For this review, take the finished solid that the model builds, in its own axes (mm). Round coordinates to 2 decimals unless told otherwise and drop trailing zeros. Order: outer loops, then holes, each group sorted by start corner. A loop starts at its lowest first (then second) coordinate and runs counter-clockwise, first axis right, second up. Notation, with made-up numbers: (83, 76) - (101, 76) arc R33 cw to (101, 114) - close; hole circle Ø4 at (-16, -25). An arc over 180 degrees is marked (long way). One line per question, with ' | ' between items.
```python
from build123d import *

# Parameters (mm, degrees)
CUT_EXTRUDE1_DEPTH = 0.8


with BuildPart() as part:
    # Sketch2 → Revolve1 (revolve)
    with BuildSketch(Plane.XY, mode=Mode.PRIVATE) as revolve1_sk:
        Polygon((0, 0), (0, 3), (0.2, 3), (1.7, 1.5), (17.75, 1.5), (18, 1.25), (18, 0), align=None)
    revolve(revolve1_sk.sketch.rotate(Axis((-2.281841559, 0, 0), (1, 0, 0)), 90), axis=Axis((-2.281841559, 0, 0), (1, 0, 0)))

    # Sketch3 → Cut-Extrude1 (cut)
    with BuildSketch(Plane.ZY):
        Polygon((0.721687836, -1.25), (1.443375673, 0), (0.721687836, 1.25), (-0.721687836, 1.25), (-1.443375673, 0), (-0.721687836, -1.25), align=None)
    extrude(amount=-CUT_EXTRUDE1_DEPTH, mode=Mode.SUBTRACT)


solid = part.part
```
(1) We need section B-B on x = 9.25. State the section outline as (y, z) points.
Output values:
outline: circle Ø3 at (0, 0)
(2) We need section A-A on z = 0. State the section outline as (x, y) points, plus the area to 3 significant figures.
Output values:
outline: (0, -3) - (0.2, -3) - (1.7, -1.5) - (17.75, -1.5) - (18, -1.25) - (18, 1.25) - (17.75, 1.5) - (1.7, 1.5) - (0.2, 3) - (0, 3) - (0, 1.25) - (0.8, 1.25) - (0.8, -1.25) - (0, -1.25) - close | area: 54.8 mm^2
(3) Mouldability with a two-part tool opening along Z and no side actions: class faces 1 (the flat face through (0, 0.6, -1.3)), 2 (the flat face through (0.8, 0, 0)), 3 (the cylindrical face through (9.84, -0.45, 1.43)) as released by +Z, released by -Z, zero draft, split by the parting line, or undercut.
Output values:
face 1: zero draft | face 2: undercut | face 3: split by the parting line
(4) Insertion check: pin 1 (3 mm diameter, centred on x = 16, z = 1.5, fed in from -Y); pin 2 (3 mm diameter, centred on x = 10, y = 1.5, fed in from -Z); pin 3 (3 mm diameter, centred on y = 0.5, z = 0, fed in from -X); pin 4 (3 mm diameter, centred on x = 10.5, y = -1.5, fed in from +Z). Each pin has a flat end and moves straight along its axis. Give the tip position at first contact, or say it passes through.
Output values:
pin 1: y = -1.5 | pin 2: z = -1.5 | pin 3: x = 0 | pin 4: z = 1.5
(5) For probe 1 along X at (y, z) = (-0.55, 0.3); probe 2 along X at (y, z) = (2.4, -0.4); probe 3 along Y at (x, z) = (16, 0.2), list the stretches that pass through material, from the lowest coordinate up. Write a range as [from, to].
Output values:
probe 1: [0.8, 18] | probe 2: [0, 0.77] | probe 3: [-1.49, 1.49]
